The listing builds one solid part. Answer for the finished solid, in the listing's coordinates (mm). A direction names the side the tool comes from. Coordinates: 2 decimals unless noted, no trailing zeros. Write each loop counter-clockwise with the first axis right and the second up, starting at its lowest first coordinate (ties: lowest second). Pieces come first, ordered by that corner, then holes.
(1) The part is cut by section C-C on x = -63.5. Determine the outline of the cut face in (y, z), plus the area to 3 significant figures.
(2) The part is cut by section B-B on y = -7.75. Give the number of separate pieces and of enclosed holes in the cut face, plus the area to 3 significant figures.
(3) The part is cut by section A-A on z = -156. Determine the outline of the cut face in (x, y), plus the area to 3 significant figures.
(4) Given P1, Ø3, axis at y = -5, z = -15, coming from the -X side; P2, Ø1, axis at y = -4, z = -67.5, coming from the -X side; P3, Ø6, axis at y = -6.5, z = 59, coming from the -X side, each flat-ended and moving along its own axis, determine where each tip first touches the part or whether it passes through.
(5) Which of the six approach directions +Z, -Z, +X, -X, +Y, -Y give full straight-line access (tool end or side, diameter ignored) to faces 4 (the cylindrical face through (73.76, -5.916, 147.865)), 5 (the flat face through (-45.421, -6, 153)), 6 (the cylindrical face through (22.456, -5.916, 73.596))?
(6) For a pull along Z with two mould halves and no side action, classify faces 1 (the cylindrical face through (-42.27, -5.916, 109.326)), 2 (the cylindrical face through (129.657, -5.916, 198.986)), 3 (the cylindrical face through (62.39, -5.92, -221.45)) as +Z half, -Z half, draft (parallel to the pull), parting line (faces both ways), or undercut.
(7) Straight lines are drawn through the part: line 1 (Z direction, x = -9, y = -8.75); line 2 (Z direction, x = 36.5, y = -0.75); line 3 (X direction, y = -6.5, z = 139). For each, find the intervals that lie inside material, in ascending order.
from build123d import *

# Parameters (mm, degrees)
F0_R     = 3.24
F0_R_2   = 5
F0_R_3   = 2.5
F0_R_4   = 19.05
F1_DEPTH = 12


with BuildPart() as f1:
    # F0 (on Front) → F1 (new body)
    with BuildSketch(Plane.XZ):
        with BuildLine():
            Line((115.360413, 205), (85.230881, 205))
            Line((85.230881, 205), (25.307446, 205))
            Line((25.307446, 205), (10.35451, 205))
            Line((10.35451, 205), (-13.005401, 205))
            Line((-13.005401, 205), (-25.421186, 205))
            ThreePointArc((-25.421186, 205), (-39.563321, 199.142136), (-45.421186, 185))
            Line((-45.421186, 185), (-45.421186, 120.10159))
            ThreePointArc((-45.421186, 120.10159), (-42.182465, 109.190149), (-33.515232, 101.81262))
            Line((-33.515232, 101.81262), (13.877641, 80.838222))
            ThreePointArc((13.877641, 80.838222), (22.544873, 73.460693), (25.783595, 62.549252))
            Line((25.783595, 62.549252), (25.783595, 57.225308))
            ThreePointArc((25.783595, 57.225308), (24.512499, 50.209031), (20.860781, 44.08459))
            Line((20.860781, 44.08459), (-88.418227, -81.298206))
            ThreePointArc((-88.418227, -81.298206), (-92.069946, -87.422647), (-93.341041, -94.438924))
            Line((-93.341041, -94.438924), (-93.341041, -135.075137))
            Line((-93.341041, -135.075137), (-93.341041, -183.041223))
            ThreePointArc((-93.341041, -183.041223), (-91.911264, -190.467313), (-87.826359, -196.831639))
            Line((-87.826359, -196.831639), (-68.18331, -217.464505))
            ThreePointArc((-68.18331, -217.464505), (-61.578084, -222.056258), (-53.697992, -223.674089))
            Line((-53.697992, -223.674089), (53.22585, -223.674089))
            ThreePointArc((53.22585, -223.674089), (62.510458, -221.388378), (69.672873, -215.053695))
            Line((69.672873, -215.053695), (102.386198, -167.7729))
            ThreePointArc((102.386198, -167.7729), (104.160024, -164.639544), (105.343296, -161.238918))
            Line((105.343296, -161.238918), (134.764535, -43.422655))
            ThreePointArc((134.764535, -43.422655), (135.210885, -41.018094), (135.360413, -38.577032))
            Line((135.360413, -38.577032), (135.360413, 185))
            ThreePointArc((135.360413, 185), (129.502549, 199.142136), (115.360413, 205))
        make_face()
        with Locations((-73.341041, -139.456751)):
            Circle(F0_R, mode=Mode.SUBTRACT)
        with Locations((-18.341041, -203.674089)):
            Circle(F0_R_2, mode=Mode.SUBTRACT)
        with Locations((-33.341041, -139.456751)):
            Circle(F0_R, mode=Mode.SUBTRACT)
        with Locations((-73.341041, -99.456751)):
            Circle(F0_R, mode=Mode.SUBTRACT)
        with Locations((-33.341041, -99.456751)):
            Circle(F0_R, mode=Mode.SUBTRACT)
        with Locations((26.658959, -203.674089)):
            Circle(F0_R_2, mode=Mode.SUBTRACT)
        with Locations((46.658959, -139.456751)):
            Circle(F0_R, mode=Mode.SUBTRACT)
        with Locations((86.658959, -139.456751)):
            Circle(F0_R, mode=Mode.SUBTRACT)
        with Locations((46.658959, -99.456751)):
            Circle(F0_R, mode=Mode.SUBTRACT)
        with Locations((86.658959, -99.456751)):
            Circle(F0_R, mode=Mode.SUBTRACT)
        with Locations((-9.692554, 134.456751)):
            Circle(F0_R_2, mode=Mode.SUBTRACT)
        with Locations((-9.692554, 179.456751)):
            Circle(F0_R_2, mode=Mode.SUBTRACT)
        with Locations((35.307446, 134.456751)):
            Circle(F0_R_2, mode=Mode.SUBTRACT)
        with Locations((65.307446, 135.886751)):
            Circle(F0_R_3, mode=Mode.SUBTRACT)
        with Locations((35.307446, 179.456751)):
            Circle(F0_R_2, mode=Mode.SUBTRACT)
        with Locations((65.307446, 183.026751)):
            Circle(F0_R_3, mode=Mode.SUBTRACT)
        with Locations((112.447446, 135.886751)):
            Circle(F0_R_3, mode=Mode.SUBTRACT)
        with Locations((88.877446, 159.456751)):
            Circle(F0_R_4, mode=Mode.SUBTRACT)
        with Locations((112.447446, 183.026751)):
            Circle(F0_R_3, mode=Mode.SUBTRACT)
    extrude(amount=F1_DEPTH)


solid = f1.part
Model answer:
1. outline: (-12, -221.11) - (0, -221.11) - (0, -52.71) - (-12, -52.71) - close
1. area: 2,020 mm2
2. separate pieces: 1
2. enclosed holes: 19
2. area: 71,900 mm2
3. outline: (-93.34, -12) - (106.65, -12) - (106.65, 0) - (-93.34, 0) - close
3. area: 2,400 mm2
4. P1: stops at x = -31.94
4. P2: stops at x = -76.83
4. P3: stops at x = 25.75
5. face 4: +Y, -Y
5. face 5: +Z, -X, +Y, -Y
5. face 6: -X, +Y, -Y
6. face 1: undercut
6. face 2: +Z half
6. face 3: -Z half
7. line 1: z = -223.67 to 9.82, 90.96 to 129.5, 139.41 to 174.5, 184.41 to 205
7. line 2: z = -223.67 to 129.6, 139.31 to 174.6, 184.31 to 205
7. line 3: x = -45.42 to -11.78, -7.6 to 33.22, 37.4 to 135.36
